from build123d import *


# Not quite as in the source:
# - a feature of the source that left no trace in its solid (it failed there, or was rolled back) is left out


with BuildPart() as f1:
    # F0 (on Front) → F1 (revolve)
    with BuildSketch(Plane.XZ):
        Polygon((-38.1, 46.1013156182), (-38.1, 0), (-38.1, -46.1013156182), (-6.35, -83.9394921831), (0, -91.5071274961), (0, 83.9394921831), (-6.35, 83.9394921831), align=None)
        Polygon((-22.676805286, 103.3970210383), (-6.35, 83.9394921831), (0, 91.5071274961), (0, 103.3970210383), align=None)
        Polygon((0, 91.5071274961), (-6.35, 83.9394921831), (0, 83.9394921831), align=None)
        Polygon((0, -91.5071274961), (-6.35, -83.9394921831), (-22.676805286, -103.3970210383), (0, -103.3970210383), align=None)
    revolve(axis=Axis((0, 0, 0), (0, 0, -1)))


solid = f1.part
Verification items for the finished model (mm, model axes). A direction names the side the tool comes from. Give positions to 0.01 mm unless a question says otherwise; leave off trailing zeros. Loops run counter-clockwise (first coordinate to the right, second up) from the corner with the lowest first, then second, coordinate; pieces in that order, holes last.
1) Sectioned sample at C-C, the plane z = 31.5. Enter the section's corners in (x, y), then the cut area to 3 significant figures.
2) Draft check along Z on faces 1 (the flat face through (0, 0, -103.397)), 2 (the conical face through (9.1, -6.9, -77.9)), 3 (the flat face through (0, 0, 103.397)). Enter one of: pulls with the +Z half, pulls with the -Z half, needs draft (parallel to the pull), parting line crosses it, or undercut.
3) Thickness scan on line 1 along Z through (x, y) = (-10.5, 1); line 2 along X through (y, z) = (-1, -31); line 3 along Z through (x, y) = (0, -14). Record the ranges inside material, lowest first.
4) Sectioned sample at A-A, the plane x = 0. Enter the section's corners in (y, z).
5) Depth check by flat-ended pin: pin 1 Ø1.5 at (x, z) = (13, -15.5) entering from -Y; pin 2 Ø6 at (y, z) = (-0.5, -65.5) entering from +X; pin 3 Ø1 at (y, z) = (21.5, -3.5) entering from -X. Enter the tip coordinate at first touch or a pass-through.
6) Set-up check for faces 4 (the cylindrical face through (30.235, -23.183, -0.645)), 5 (the conical face through (1.942, -8.744, 87.046)): record each of +Z, -Z, +X, -X, +Y, -Y from which the full face is reachable in a straight line by a thin tool's end or side.
7) Sectioned sample at D-D, the plane y = -15. Count the separate pieces of the cut face and the enclosed holes in it, then the cut area to 3 significant figures.
Answers:
1. outline: circle Ø76.2 at (0, 0)
1. area: 4,560 mm2
2. face 1: pulls with the -Z half
2. face 2: undercut
2. face 3: pulls with the +Z half
3. line 1: z = -103.4 to -88.94, -78.94 to 78.94, 88.94 to 103.4
3. line 2: x = -38.09 to 38.09
3. line 3: z = -103.4 to -93.06, -74.82 to 74.82, 93.06 to 103.4
4. outline: (-38.1, -46.1) - (-6.35, -83.94) - (-22.68, -103.4) - (22.68, -103.4) - (6.35, -83.94) - (38.1, -46.1) - (38.1, 46.1) - (6.35, 83.94) - (22.68, 103.4) - (-22.68, 103.4) - (-6.35, 83.94) - (-38.1, 46.1) - close
5. pin 1: stops at y = -36.08
5. pin 2: stops at x = 24.34
5. pin 3: stops at x = -31.79
6. face 4: +Z, -Z
6. face 5: none
7. separate pieces: 3
7. enclosed holes: 0
7. area: 9,190 mm2
